from build123d import *

# Parameters (mm, degrees)
SKETCH3_R               = 3
BOSS_EXTRUDE1_DEPTH     = 19
SKETCH4_R               = 0.75
CUT_EXTRUDE1_DEPTH      = 4
CUT_EXTRUDE1_DEPTH_BACK = 4
CHAMFER1_SIZE           = 0.25


with BuildPart() as part:
    # Sketch3 → Boss-Extrude1 (new body)
    with BuildSketch(Plane.XY):
        Circle(SKETCH3_R)
    extrude(amount=BOSS_EXTRUDE1_DEPTH)

    # Sketch4 → Cut-Extrude1 (cut, two sides)
    with BuildSketch(Plane(origin=(0, 0, 0), x_dir=(0, 0, -1), z_dir=(1, 0, 0))) as cut_extrude1_sk:
        with Locations((-2.5, 0)):
            Circle(SKETCH4_R)
        with Locations((-16.5, 0)):
            Circle(SKETCH4_R)
    extrude(amount=CUT_EXTRUDE1_DEPTH, mode=Mode.SUBTRACT)
    extrude(cut_extrude1_sk.sketch, amount=-CUT_EXTRUDE1_DEPTH_BACK, mode=Mode.SUBTRACT)

    # Chamfer1
    chamfer1_edges = [part.edges().sort_by_distance(p)[0] for p in [
        (-3, 0, 0),
        (-3, 0, 19),
    ]]
    chamfer(chamfer1_edges, length=CHAMFER1_SIZE)


solid = part.part
Here's how the part is built. I have some questions about the finished solid (model axes, mm). Give positions to 0.01 mm unless a question says otherwise; leave off trailing zeros. Loops run counter-clockwise (first coordinate to the right, second up) from the corner with the lowest first, then second, coordinate; pieces in that order, holes last. Notation, with made-up numbers: (87, 75.25) -> (104, 75.25) arc R14 cw to (104, 95.25) -> close; hole circle Ø8 at (-4.5, -20). An arc over 180 degrees is marked (long way). One line per item, written item: value.
Q1. Suppose I cut it at B-B on z = 2. Please give me the cut outline in (x, y), then the cut area to 3 significant figures.
Answers follow:
outline: (-2.95, -0.56) arc R3 ccw to (2.95, -0.56) -> close; (-2.95, 0.56) -> (2.95, 0.56) arc R3 ccw to start
area: 21.6 mm^2
Q2. Suppose I cut it at D-D on x = -2. State how many separate pieces and enclosed holes the cut face has, then the cut area to 3 significant figures.
Answers follow:
separate pieces: 1
enclosed holes: 2
area: 81.3 mm^2
Q3. If I drill on line 1 along Z through (x, y) = (1.2, 0); line 2 along Y through (x, z) = (1.2, 2.5); line 3 along Z through (x, y) = (-1.5, 0.5), over which ranges is the centre line in solid material (lowest first)?
Answers follow:
line 1: 0 to 1.75, 3.25 to 15.75, 17.25 to 19
line 2: -2.75 to -0.75, 0.75 to 2.75
line 3: 0 to 1.94, 3.06 to 15.94, 17.06 to 19
Q4. I'm going to push flat-ended pins straight in: pin 1 Ø1.5 at (y, z) = (-1, 2.5) entering from -X; pin 2 Ø1.5 at (y, z) = (2, 10.5) entering from +X; pin 3 Ø1.5 at (y, z) = (1, 8.5) entering from +X. Where does each tip first touch, or does it pass through?
Answers follow:
pin 1: x = -2.96
pin 2: x = 2.73
pin 3: x = 2.99
Q5. Suppose I cut it at C-C on z = 14. Please give me the cut outline in (x, y), then the cut area to 3 significant figures.
Answers follow:
outline: circle Ø6 at (0, 0)
area: 28.3 mm^2
Q6. Suppose I cut it at A-A on y = 0. Please give me the cut outline in (x, z).
Answers follow:
outline: (-3, 0.25) -> (-2.75, 0) -> (2.75, 0) -> (3, 0.25) -> (3, 1.75) -> (-3, 1.75) -> close; (-3, 3.25) -> (3, 3.25) -> (3, 15.75) -> (-3, 15.75) -> close; (-3, 17.25) -> (3, 17.25) -> (3, 18.75) -> (2.75, 19) -> (-2.75, 19) -> (-3, 18.75) -> close
